Source: three-view drawing plus pictorial views. Frame: mm from the lowest corner of the part. A direction names the side the tool comes from. Round coordinates to 2 decimals unless told otherwise and drop trailing zeros. Order: outer loops, then holes, each group sorted by start corner. A loop starts at its lowest first (then second) coordinate and runs counter-clockwise, first axis right, second up. Notation, with made-up numbers: M 3,51.25 L 33,51.25 A8 cw 33,59.25 Z; hole C 70.25,-26.5 d6. An arc over 180 degrees is marked long. Return JSON: item names as keys, results as strings. Group by question number.
Q1. Contact query for flat-ended pins moving along their axis: pin 1 (10 mm diameter, centred on x = 20.5, z = 32.5, fed in from -Y); pin 2 (8 mm diameter, centred on x = 12.5, z = 48, fed in from +Y). Output: stop coordinate, or through.
Q2. Cut plane A-A on y = 6.75. Output: boundary loops of the cut face in (x, z), and give its area (3 significant figures).
Q3. Cut plane B-B on x = 8. Output: boundary loops of the cut face in (y, z), and give its area (3 significant figures).
Q4. Cut plane C-C on z = 32. Output: boundary loops of the cut face in (x, y).
Q5. Mould query, pull axis Z, two halves, no side actions, for the marked faces 1, 2 and 3. Classes: released by +Z, released by -Z, zero draft, split by the parting line, or undercut.
Q6. Ray query, probe 1 along Z at (x, y) = (23, 14); probe 2 along X at (y, z) = (5, 9); probe 3 along Z at (x, y) = (2, 9.75). Return the intervals inside material, ascending.
Q7. Access query for the marked faces 4 and 5. Directions: +Z, -Z, +X, -X, +Y, -Y. A direction counts if a zero-diameter tool reaches every point of the face in a straight line with its end or side. Return the directions, or none.
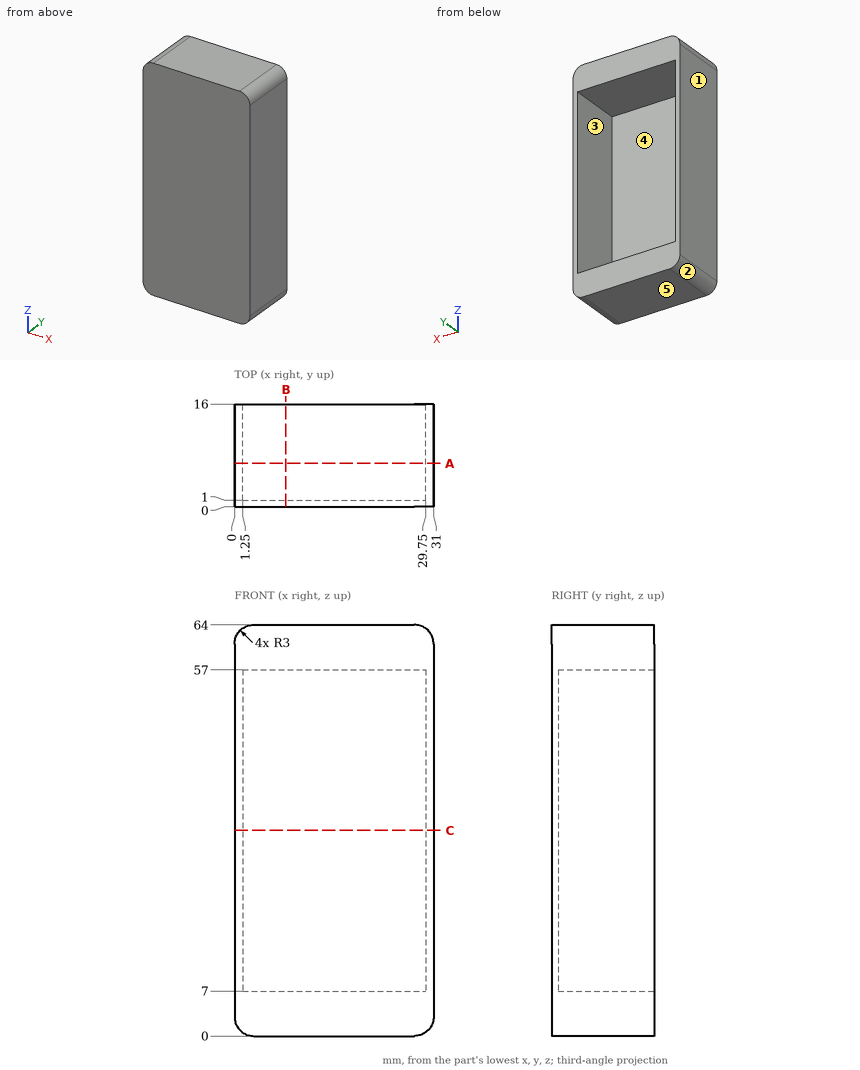
Result sheet:
{
 "1": {"pin 1": "stops at y = 0", "pin 2": "stops at y = 1"},
 "2": {"outline": "M 0,3 A3 ccw 3,0 L 28,0 A3 ccw 31,3 L 31,61 A3 ccw 28,64 L 3,64 A3 ccw 0,61 Z; hole M 1.25,7 L 29.75,7 L 29.75,57 L 1.25,57 Z", "area": "551 mm²"},
 "3": {"outline": "M 0,0 L 16,0 L 16,7 L 1,7 L 1,57 L 16,57 L 16,64 L 0,64 Z", "area": "274 mm²"},
 "4": {"outline": "M 0,0 L 31,0 L 31,16 L 29.75,16 L 29.75,1 L 1.25,1 L 1.25,16 L 0,16 Z"},
 "5": {"face 1": "zero draft", "face 2": "released by -Z", "face 3": "undercut"},
 "6": {"probe 1": "z = 0 to 7, 57 to 64", "probe 2": "x = 0 to 1.25, 29.75 to 31", "probe 3": "z = 0.17 to 7, 57 to 63.83"},
 "7": {"face 4": "+Y", "face 5": "-Z, +X, -X, +Y, -Y"}
}
